```python
from build123d import *

# Parameters (mm, degrees)
SKETCH1_W           = 68
SKETCH1_H           = 104
SKETCH1_W_2         = 26
SKETCH1_H_2         = 26
BOSS_EXTRUDE1_DEPTH = 4
FILLET1_R           = 5
CUT_EXTRUDE1_DEPTH  = 3
FILLET2_R           = 1.5
SKETCH4_R           = 2.5
BOSS_EXTRUDE2_DEPTH = 5
SKETCH5_R           = 1.5
CUT_EXTRUDE2_DEPTH  = 63.777384463


with BuildPart() as part:
    # Sketch1 → Boss-Extrude1 (new body)
    with BuildSketch(Plane(origin=(0, 0, 0), x_dir=(1, 0, 0), z_dir=(0, 1, 0))):
        Rectangle(SKETCH1_W, SKETCH1_H)
        Rectangle(SKETCH1_W_2, SKETCH1_H_2, mode=Mode.SUBTRACT)
    extrude(amount=BOSS_EXTRUDE1_DEPTH)

    # Fillet1
    fillet1_edges = [part.edges().sort_by_distance(p)[0] for p in [
        (34, 2, 52),
        (-34, 2, 52),
        (-34, 2, -52),
        (34, 2, -52),
    ]]
    fillet(fillet1_edges, radius=FILLET1_R)

    # Sketch3 → Cut-Extrude1 (cut)
    with BuildSketch(Plane(origin=(0, 4, 0), x_dir=(1, 0, 0), z_dir=(0, 1, 0))):
        with BuildLine():
            Line((29, 51.5), (-29, 51.5))
            ThreePointArc((-29, 51.5), (-32.181980515, 50.181980515), (-33.5, 47))
            Line((-33.5, 47), (-33.5, -47))
            ThreePointArc((-33.5, -47), (-32.181980515, -50.181980515), (-29, -51.5))
            Line((-29, -51.5), (29, -51.5))
            ThreePointArc((29, -51.5), (32.181980515, -50.181980515), (33.5, -47))
            Line((33.5, -47), (33.5, 47))
            ThreePointArc((33.5, 47), (32.181980515, 50.181980515), (29, 51.5))
        make_face()
        with BuildLine():
            Line((-28.5, -32.5), (-28.5, 32.5))
            ThreePointArc((-28.5, 32.5), (-23.5, 37.5), (-18.5, 32.5))
            Line((-18.5, 32.5), (-18.5, -32.5))
            ThreePointArc((-18.5, -32.5), (-23.5, -37.5), (-28.5, -32.5))
        make_face(mode=Mode.SUBTRACT)
        with BuildLine():
            Line((18.5, -32.5), (18.5, 32.5))
            ThreePointArc((18.5, 32.5), (23.5, 37.5), (28.5, 32.5))
            Line((28.5, 32.5), (28.5, -32.5))
            ThreePointArc((28.5, -32.5), (23.5, -37.5), (18.5, -32.5))
        make_face(mode=Mode.SUBTRACT)
    extrude(amount=-CUT_EXTRUDE1_DEPTH, mode=Mode.SUBTRACT)

    # Fillet2
    fillet2_edges = [part.edges().sort_by_distance(p)[0] for p in [
        (23.5, 4, -37.5),
        (28.5, 4, 0),
        (23.5, 4, 37.5),
        (23.5, 1, -37.5),
        (28.5, 1, 0),
        (23.5, 1, 37.5),
        (-23.5, 4, -37.5),
        (-18.5, 4, 0),
        (-23.5, 4, 37.5),
        (-23.5, 1, -37.5),
        (-18.5, 1, 0),
        (-23.5, 1, 37.5),
        (18.5, 4, 0),
        (18.5, 1, 0),
        (-28.5, 4, 0),
        (-28.5, 1, 0),
    ]]
    fillet(fillet2_edges, radius=FILLET2_R - 0.0001)  # a hair under: the kernel refuses the full size

    # Sketch4 → Boss-Extrude2 (add)
    with BuildSketch(Plane.XZ):
        with Locations(Location((-27, 45, 0), (0, 0, 270))):
            Circle(SKETCH4_R)
        with Locations(Location((27, 45, 0), (0, 0, 270))):
            Circle(SKETCH4_R)
        with Locations(Location((27, -45, 0), (0, 0, 270))):
            Circle(SKETCH4_R)
        with Locations(Location((-27, -45, 0), (0, 0, 270))):
            Circle(SKETCH4_R)
    extrude(amount=BOSS_EXTRUDE2_DEPTH)

    # Sketch5 → Cut-Extrude2 (cut, through all)
    with BuildSketch(Plane.XZ.offset(5)):
        with Locations(Location((-27, 45, 0), (0, 0, 270))):
            Circle(SKETCH5_R)
        with Locations(Location((27, 45, 0), (0, 0, 270))):
            Circle(SKETCH5_R)
        with Locations(Location((27, -45, 0), (0, 0, 270))):
            Circle(SKETCH5_R)
        with Locations(Location((-27, -45, 0), (0, 0, 270))):
            Circle(SKETCH5_R)
    extrude(amount=-CUT_EXTRUDE2_DEPTH, mode=Mode.SUBTRACT)


solid = part.part
```
The listing builds one solid part. Answer for the finished solid, in the listing's coordinates (mm). A direction names the side the tool comes from. Coordinates: 2 decimals unless noted, no trailing zeros. Order: outer loops, then holes, each group sorted by start corner. A loop starts at its lowest first (then second) coordinate and runs counter-clockwise, first axis right, second up. Notation, with made-up numbers: M 27.25,62.25 L 62.25,62.25 A9 cw 62.25,73.25 Z; hole C 27,63 d4. An arc over 180 degrees is marked long. Answer as a JSON object with one key per item and string values. Group by question number.
1. Flat-ended cylindrical pins translate along their axes: P1, Ø6, axis at x = 27, z = 16.5, coming from the -Y side; P2, Ø4, axis at x = 27, z = 45, coming from the +Y side. Find the tip coordinate at first contact, or state that the pin passes through.
2. Determine the mould class of faces 3 (the flat face through (-24, 4, -1)), 4 (the cylindrical face through (-33, 2, 50)), 5 (the cylindrical face through (-24.89, -2.46, -46.34)) for opening direction X: released by +X, released by -X, zero draft, split by the parting line, or undercut.
3. Section B-B on x = -5 is taken. Write down the section's boundary in (y, z), then the cut area to 3 significant figures.
4. Section A-A on z = 45 is taken. Write down the section's boundary in (x, y), then the cut area to 3 significant figures.
5. Straight lines are drawn through the part: line 1 (X direction, y = -3.45, z = -45); line 2 (X direction, y = -2.75, z = -45.5); line 3 (Z direction, x = 3, y = 2.5). For each, find the intervals that lie inside material, in ascending order.
6. A tool of negligible diameter and unlimited length cuts with its end or side. For faces 1 (the cylindrical face through (-32.147, 2.521, -50.217)), 2 (the cylindrical face through (28.01, -2.04, 46.11)), from which of +Z, -Z, +X, -X, +Y, -Y can it reach the whole face along a straight path? Write none if from no direction.
Values follow:
{
 "1": {"P1": "y = 0", "P2": "y = 1"},
 "2": {"face 3": "zero draft", "face 4": "released by -X", "face 5": "undercut"},
 "3": {"outline": "M 0,-52 L 4,-52 L 4,-51.5 L 1,-51.5 L 1,-13 L 0,-13 Z; M 0,13 L 1,13 L 1,51.5 L 4,51.5 L 4,52 L 0,52 Z", "area": "81.0 mm2"},
 "4": {"outline": "M -34,0 L -29.5,0 L -29.5,-5 L -28.5,-5 L -28.5,1 L -33.5,1 L -33.5,4 L -34,4 Z; M -25.5,-5 L -24.5,-5 L -24.5,0 L 24.5,0 L 24.5,-5 L 25.5,-5 L 25.5,1 L -25.5,1 Z; M 28.5,-5 L 29.5,-5 L 29.5,0 L 34,0 L 34,4 L 33.5,4 L 33.5,1 L 28.5,1 Z", "area": "85.0 mm2"},
 "5": {"line 1": "-29.5 to -28.5, -25.5 to -24.5, 24.5 to 25.5, 28.5 to 29.5", "line 2": "-29.45 to -28.41, -25.59 to -24.55, 24.55 to 25.59, 28.41 to 29.45", "line 3": "-52 to -51.5, 51.5 to 52"},
 "6": {"face 1": "+Y", "face 2": "+Y, -Y"}
}
